Autodesk Inventor part; units mm, degrees
ref_plane "YZ Plane" through (0, 0, 0) normal (1, 0, 0) x (0, 1, 0)
ref_plane "XZ Plane" through (0, 0, 0) normal (0, 1, 0) x (-1, 0, 0)
ref_plane "XY Plane" through (0, 0, 0) normal (0, 0, 1) x (1, 0, 0)
sketch "Boceto1" plane through (0, 0, 0) normal (0, 1, 0) x (-1, 0, 0)
  line L0 (-50, 50) -> (50, 50)
  line L1 (50, 50) -> (50, -50)
  line L2 (50, -50) -> (-50, -50)
  line L3 (-50, -50) -> (-50, 50)
  line L4 (-50, 50) -> (50, -50) construction
  line L5 (50, 50) -> (-50, -50) construction
  line L6 (25, 53.18) -> (-25, 53.18)
  line L7 (-25, 53.18) -> (-25, 50)
  line L8 (-25, 50) -> (25, 50)
  line L9 (25, 50) -> (25, 53.18)
  line L10 (25, -50) -> (-25, -50)
  line L11 (-25, -50) -> (-25, -53.18)
  line L12 (-25, -53.18) -> (25, -53.18)
  line L13 (25, -53.18) -> (25, -50)
  line L14 (53.18, 25) -> (50, 25)
  line L15 (50, 25) -> (50, -25)
  line L16 (50, -25) -> (53.18, -25)
  line L17 (53.18, -25) -> (53.18, 25)
  line L18 (-50, 25) -> (-53.18, 25)
  line L19 (-53.18, 25) -> (-53.18, -25)
  line L20 (-53.18, -25) -> (-50, -25)
  line L21 (-50, -25) -> (-50, 25)
  point P0 (0, 0)
  dimension "d0" = 100
  dimension "d1" = 100
  dimension "d2" = 3.18
  dimension "d3" = 3.18
  dimension "d4" = 50
  dimension "d5" = 25
  dimension "d6" = 25
  dimension "d7" = 25
extrude "Extrusión1" add sketch "Boceto1" along normal blind 3.18
properties part number "BASE_FONDO"
Verification items for the finished model (mm, model axes). A direction names the side the tool comes from. Give positions to 0.01 mm unless a question says otherwise; leave off trailing zeros. Loops run counter-clockwise (first coordinate to the right, second up) from the corner with the lowest first, then second, coordinate; pieces in that order, holes last. Notation, with made-up numbers: (4, 77) - (14, 77) arc R27 ccw to (14, 99) - close; hole circle Ø11 at (-8, -19). An arc over 180 degrees is marked (long way). Write each question's results on one line, items separated by ' | '.
1) Sectioned sample at A-A on y = 1.55. Record the boundary of the cut face in (x, z).
Solution:
outline: (-53.18, -25) - (-50, -25) - (-50, -50) - (-25, -50) - (-25, -53.18) - (25, -53.18) - (25, -50) - (50, -50) - (50, -25) - (53.18, -25) - (53.18, 25) - (50, 25) - (50, 50) - (25, 50) - (25, 53.18) - (-25, 53.18) - (-25, 50) - (-50, 50) - (-50, 25) - (-53.18, 25) - close
2) Tool access check on faces 4 (the flat face through (-38, 2, -50)), 5 (the flat face through (-37, 2, 50)), 6 (the flat face through (50, 2, 37)), 7 (the flat face through (37, 2, -50)). Record the directions out of +Z, -Z, +X, -X, +Y, -Y that give a thin tool (end or side, any length) a straight path to the whole face; none if there is none.
Solution:
face 4: -Z, -X, +Y, -Y | face 5: +Z, -X, +Y, -Y | face 6: +Z, +X, +Y, -Y | face 7: -Z, +X, +Y, -Y
3) Sectioned sample at B-B on z = -44. Record the boundary of the cut face in (x, y).
Solution:
outline: (-50, 0) - (50, 0) - (50, 3.18) - (-50, 3.18) - close
4) Sectioned sample at C-C on x = -34. Record the boundary of the cut face in (y, z).
Solution:
outline: (0, -50) - (3.18, -50) - (3.18, 50) - (0, 50) - close
5) Material ranges on L1, parallel to Z at x = 34, y = 2.75, recorded low to high. Write a range as from..to.
Solution:
L1: -50..50
6) Mould release check, pull along Y, two halves, no side actions. Record for faces 1 (the flat face through (1, 0, 1)), 2 (the flat face through (-25, 2, 52)), 3 (the flat face through (1, 3.18, 1)): pulls with the +Y half, pulls with the -Y half, needs draft (parallel to the pull), parting line crosses it, or undercut.
Solution:
face 1: pulls with the -Y half | face 2: needs draft | face 3: pulls with the +Y half
7) Depth check by flat-ended pin: P1, Ø1.6, axis at y = 1.5, z = -31.5, coming from the -X side; P2, Ø4, axis at x = -19.5, z = -29.5, coming from the -Y side; P3, Ø1, axis at y = 1, z = 51, coming from the -X side; P4, Ø1, axis at x = 52, y = 1, coming from the -Z side. Enter the tip coordinate at first touch or a pass-through.
Solution:
P1: x = -50 | P2: y = 0 | P3: x = -25 | P4: z = -25
